Geometry check sheet. Reference: drawing and pictorial views, mm from the part's lowest x, y, z. A direction names the side the tool comes from. Round coordinates to 2 decimals unless told otherwise and drop trailing zeros. Write each loop counter-clockwise with the first axis right and the second up, starting at its lowest first coordinate (ties: lowest second). Pieces come first, ordered by that corner, then holes. Notation, with made-up numbers: (28.5, -9.75) -> (50.5, -9.75) arc R18 cw to (50.5, 23.25) -> close; hole circle Ø7 at (19, -39.5). An arc over 180 degrees is marked (long way). Write item = value, one per line.
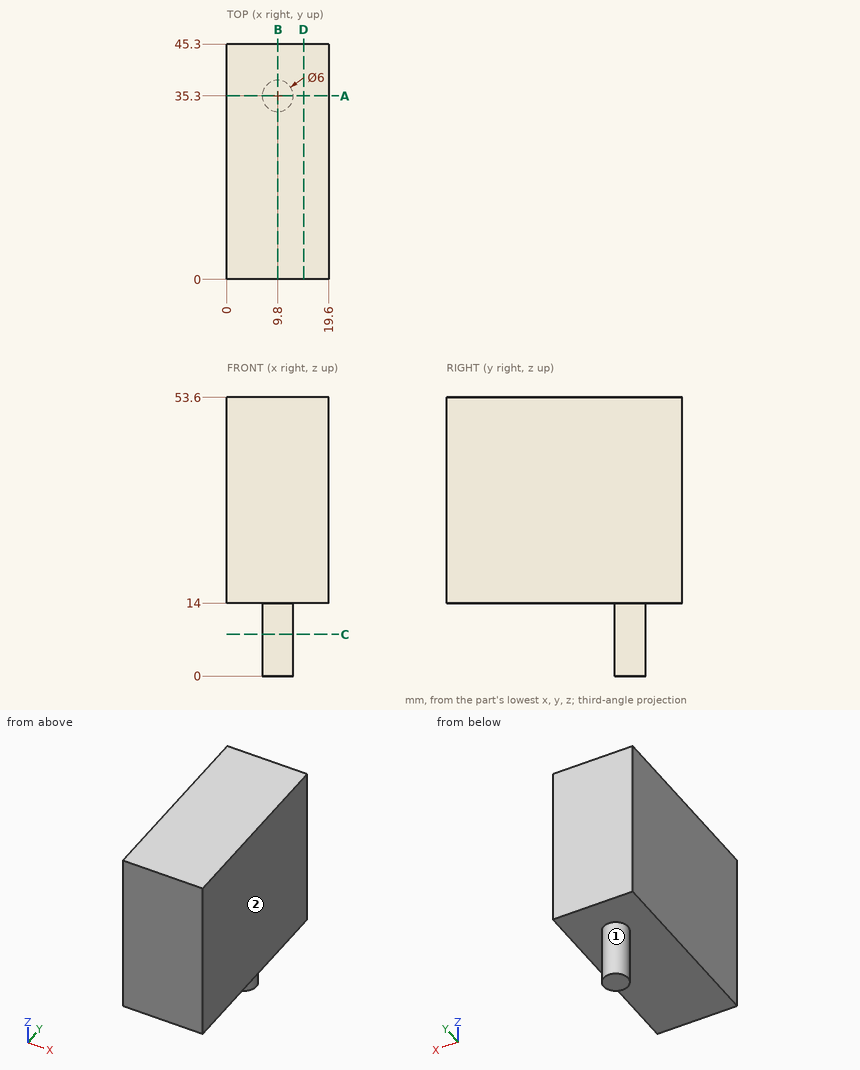
(1) Access from +Z, -Z, +X, -X, +Y, -Y to the whole of each face (thin tool, end or side, straight path). Record for the marked faces 1 and 2.
Worked answers:
face_1 = -Z
face_2 = +Z, -Z, +X, +Y, -Y
(2) Go/stop test with flat-tipped pins: P1, Ø6, axis at y = 23, z = 19, coming from the -X side; P2, Ø4, axis at x = 3, y = 12.5, coming from the -Z side. Record where each tip stops, or that it passes through.
Worked answers:
P1 = 0
P2 = 14
(3) Sectioned sample at D-D on x = 14.75. Enter the section's corners in (y, z), then the cut area to 3 significant figures.
Worked answers:
outline = (0, 14) -> (45.3, 14) -> (45.3, 53.6) -> (0, 53.6) -> close
area = 1,790 mm²
(4) Sectioned sample at B-B on x = 9.8. Enter the section's corners in (y, z).
Worked answers:
outline = (0, 14) -> (32.3, 14) -> (32.3, 0) -> (38.3, 0) -> (38.3, 14) -> (45.3, 14) -> (45.3, 53.6) -> (0, 53.6) -> close
(5) Material ranges on L1, parallel to Z at x = 2, y = 7.5; L2, parallel to Y at x = 10.5, z = 3.5, recorded low to high. Write a range as [from, to].
Worked answers:
L1 = [14, 53.6]
L2 = [32.38, 38.22]
(6) Sectioned sample at A-A on y = 35.3. Enter the section's corners in (x, z).
Worked answers:
outline = (0, 14) -> (6.8, 14) -> (6.8, 0) -> (12.8, 0) -> (12.8, 14) -> (19.6, 14) -> (19.6, 53.6) -> (0, 53.6) -> close
(7) Sectioned sample at C-C on z = 8. Enter the section's corners in (x, y), then the cut area to 3 significant figures.
Worked answers:
outline = circle Ø6 at (9.8, 35.3)
area = 28.3 mm²
